Model file for the job. Use its own axes, mm. A direction names the side the tool comes from. Coordinates: 2 decimals unless noted, no trailing zeros. Order: outer loops, then holes, each group sorted by start corner. A loop starts at its lowest first (then second) coordinate and runs counter-clockwise, first axis right, second up. Notation, with made-up numbers: M 7,-18.75 L 45,-18.75 A34 cw 45,20.25 Z; hole C 65.5,79.5 d9. An arc over 180 degrees is marked long. Return JSON: item names as keys, results as strings.
```python
from build123d import *
from build123d.topology import SkipClean

# Parameters (mm, degrees)
SKETCH1_R             = 10
SKETCH1_R_2           = 3
BOSS_EXTRUDE1_DEPTH   = 7.5
BOSS_EXTRUDE1_2_DEPTH = 7.5
BOSS_EXTRUDE1_3_DEPTH = 7.5
BOSS_EXTRUDE1_4_DEPTH = 7.5
BOSS_EXTRUDE2_DEPTH   = 7.5
SKETCH3_R             = 3
CUT_EXTRUDE1_DEPTH    = 15
FILLET1_R             = 5


with BuildPart() as part:
    # Sketch1 → Boss-Extrude1 (new, symmetric)
    with BuildSketch(Plane.XY):
        with Locations((-600, 0)):
            Circle(SKETCH1_R)
        with Locations((-600, 0)):
            Circle(SKETCH1_R_2, mode=Mode.SUBTRACT)
    extrude(amount=BOSS_EXTRUDE1_DEPTH, both=True)



with BuildPart() as body_2:
    # Sketch1 → Boss-Extrude1 2 (new, symmetric)
    with BuildSketch(Plane.XY):
        with Locations((-200, -300)):
            Circle(SKETCH1_R)
        with Locations((-200, -300)):
            Circle(SKETCH1_R_2, mode=Mode.SUBTRACT)
    extrude(amount=BOSS_EXTRUDE1_2_DEPTH, both=True)


with BuildPart() as body_3:
    # Sketch1 → Boss-Extrude1 3 (new, symmetric)
    with BuildSketch(Plane.XY):
        with Locations((200, -300)):
            Circle(SKETCH1_R)
        with Locations((200, -300)):
            Circle(SKETCH1_R_2, mode=Mode.SUBTRACT)
    extrude(amount=BOSS_EXTRUDE1_3_DEPTH, both=True)


with BuildPart() as body_4:
    # Sketch1 → Boss-Extrude1 4 (new, symmetric)
    with BuildSketch(Plane.XY):
        with Locations((600, 0)):
            Circle(SKETCH1_R)
        with Locations((600, 0)):
            Circle(SKETCH1_R_2, mode=Mode.SUBTRACT)
    extrude(amount=BOSS_EXTRUDE1_4_DEPTH, both=True)


with BuildPart() as part_1:
    add(part.part)

    add(body_2.part)  # Boss-Extrude2 merges body 2

    add(body_3.part)  # Boss-Extrude2 merges body 3

    add(body_4.part)  # Boss-Extrude2 merges body 4
    # Sketch2 → Boss-Extrude2 (add, symmetric)
    with BuildSketch(Plane.XY):
        Polygon((200, -307.5), (202.5, -307.5), (204.5, -306), (622.5, 7.5), (-622.5, 7.5), (-204.5, -306), (-202.5, -307.5), (-200, -307.5), align=None)
        Polygon((201.842585459, -289.243060906), (577.5, -7.5), (14.013878189, -7.5), align=None, mode=Mode.SUBTRACT)
        Polygon((-577.5, -7.5), (-201.842585459, -289.243060906), (-14.013878189, -7.5), align=None, mode=Mode.SUBTRACT)
        Polygon((-185.986121811, -292.5), (185.986121811, -292.5), (0, -13.520817283), align=None, mode=Mode.SUBTRACT)
    extrude(amount=BOSS_EXTRUDE2_DEPTH, both=True)

    # Sketch3 → Cut-Extrude1 (cut, symmetric)
    with SkipClean():  # the faces are left unmerged after this step: merging them gives an invalid solid
        with BuildSketch(Plane.XY):
            with Locations((-600, 0)):
                Circle(SKETCH3_R)
            with Locations((-200, -300)):
                Circle(SKETCH3_R)
            with Locations((200, -300)):
                Circle(SKETCH3_R)
            with Locations((600, 0)):
                Circle(SKETCH3_R)
            with BuildLine():
                Line((605.772412725, 8.165736423), (623.676739049, 10.899071484))
                Line((623.676739049, 10.899071484), (625.286418453, -4.2155453))
                Line((625.286418453, -4.2155453), (609.468772967, -3.215950638))
                ThreePointArc((609.468772967, -3.215950638), (609.511000758, 3.088829), (605.772412725, 8.165736423))
            make_face()
            with BuildLine():
                Line((-625.286418453, -4.2155453), (-609.468772967, -3.215950638))
                ThreePointArc((-609.468772967, -3.215950638), (-609.511000758, 3.088829), (-605.772412725, 8.165736423))
                Line((-605.772412725, 8.165736423), (-623.676739049, 10.899071484))
                Line((-623.676739049, 10.899071484), (-625.286418453, -4.2155453))
            make_face()
        extrude(amount=CUT_EXTRUDE1_DEPTH, both=True, mode=Mode.SUBTRACT)

    # Fillet1
    fillet1_edges = [part_1.edges().sort_by_distance(p)[0] for p in [
        (0, -13.520817283, 0),
        (-185.986121811, -292.5, 0),
        (185.986121811, -292.5, 0),
        (14.013878189, -7.5, 0),
        (201.842585459, -289.243060906, 0),
        (577.5, -7.5, 0),
        (-577.5, -7.5, 0),
        (-201.842585459, -289.243060906, 0),
        (-14.013878189, -7.5, 0),
    ]]
    fillet(fillet1_edges, radius=FILLET1_R)


solid = part_1.part
```
Item 1: Drop flat-ended pins along their axis: pin 1 Ø8 at (y, z) = (-59.5, -3.5) entering from +X; pin 2 Ø3.5 at (x, y) = (-600, 0) entering from +Z; pin 3 Ø8 at (y, z) = (-51, -5.5) entering from -X; pin 4 Ø4 at (y, z) = (-176.5, -1.5) entering from +X. Give the stop position or say it passes through.
Check result:
{"pin 1": "stops at x = 538.5", "pin 2": "passes through", "pin 3": "stops at x = -549.83", "pin 4": "stops at x = 379.83"}
Item 2: Saw through at B-B (y = -165). Write the cut outline in (x, z), and give its area (3 significant figures).
Check result:
{"outline": "M -392.5,-7.5 L -367.5,-7.5 L -367.5,7.5 L -392.5,7.5 Z; M -119.01,-7.5 L -100.99,-7.5 L -100.99,7.5 L -119.01,7.5 Z; M 100.99,-7.5 L 119.01,-7.5 L 119.01,7.5 L 100.99,7.5 Z; M 367.5,-7.5 L 392.5,-7.5 L 392.5,7.5 L 367.5,7.5 Z", "area": "1,290 mm2"}
Item 3: Saw through at A-A (z = -2.25). Count the separate pieces of the cut face and the enclosed holes in it, and give its area (3 significant figures).
Check result:
{"separate pieces": "1", "enclosed holes": "7", "area": "49,300 mm2"}
Item 4: Pull direction X, two halves, no side cores. Call faces 1 (the flat face through (-388.3, -149.4, 0.1)), 2 (the flat face through (-48, -78, -7.5)), 3 (the flat face through (-407.226, -153.956, 0.105)): +X half, -X half, draft (parallel to the pull), parting line (faces both ways), or undercut.
Check result:
{"face 1": "undercut", "face 2": "draft", "face 3": "-X half"}
Item 5: Saw through at C-C (x = 238). Write the cut outline in (y, z) (3 decimals), and give its area (3 significant figures).
Check result:
{"outline": "M -280.875,-7.5 L -262.125,-7.5 L -262.125,7.5 L -280.875,7.5 Z; M -7.5,-7.5 L 7.5,-7.5 L 7.5,7.5 L -7.5,7.5 Z", "area": "506 mm2"}
Item 6: 3-axis set-ups, long thin cutter, end or side, ignore diameter. For faces 4 (the flat face through (-91.246, -150.389, 0.105)), 5 (the flat face through (-48, -78, 7.5)): which of +Z, -Z, +X, -X, +Y, -Y reach the whole face in a straight line?
Check result:
{"face 4": "+Z, -Z", "face 5": "+Z, +X, -X, +Y, -Y"}
Item 7: Wall check: line 1 (Y direction, x = 200, z = -1); line 2 (X direction, y = 0, z = 1); line 3 (X direction, y = -84.5, z = 3). Give the ranges that are in metal, low to high.
Check result:
{"line 1": "y = -310 to -303, -297 to -286.02, -7.5 to 7.5", "line 2": "x = -610 to -603, -597 to 597, 603 to 610", "line 3": "x = -499.83 to -474.83, -65.35 to -47.32, 47.32 to 65.35, 474.83 to 499.83"}
Item 8: Saw through at D-D (x = -38). Write the cut outline in (y, z).
Check result:
{"outline": "M -307.5,-7.5 L -292.5,-7.5 L -292.5,7.5 L -307.5,7.5 Z; M -70.52,-7.5 L -43.48,-7.5 L -43.48,7.5 L -70.52,7.5 Z; M -7.5,-7.5 L 7.5,-7.5 L 7.5,7.5 L -7.5,7.5 Z"}
